Check sheet for the drawn part. Datum: minimum x, y, z corner. Units: mm. A direction names the side the tool comes from. Give positions to 0.01 mm unless a question says otherwise; leave off trailing zeros. Order: outer loops, then holes, each group sorted by start corner. A loop starts at its lowest first (then second) coordinate and runs counter-clockwise, first axis right, second up. Notation, with made-up numbers: M 41.5,-15 L 98.5,-15 A20 cw 98.5,0 Z; hole C 12.25,89.5 d5. An arc over 180 degrees is marked long. Answer as CSV lines item,"result". Start each with the question number.
Q1. Section check C-C, the plane x = 14.25. Record the boundary of the cut face in (y, z).
Q2. Section check B-B, the plane z = 13.5. Record the boundary of the cut face in (x, y).
Q3. Set-up check for the marked faces 1 and 2: record each of +Z, -Z, +X, -X, +Y, -Y from which the full face is reachable in a straight line by a thin tool's end or side.
Q4. Section check A-A, the plane y = 4. Record the boundary of the cut face in (x, z), then the cut area to 3 significant figures.
Q5. Go/stop test with flat-tipped pins: pin 1 (1 mm diameter, centred on x = 8.5, y = 1, fed in from -Z); pin 2 (2 mm diameter, centred on y = 1, z = 8.5, fed in from -X); pin 3 (6 mm diameter, centred on x = 18, y = 10, fed in from -Z); pin 4 (1.6 mm diameter, centred on y = 19, z = 14, fed in from -X). Record where each tip stops, or that it passes through.
Q6. Thickness scan on line 1 (X direction, y = 7.25, z = 56.5); line 2 (X direction, y = 11, z = 83). Record the ranges inside material, lowest first.
Q7. Section check D-D, the plane z = 25. Record the boundary of the cut face in (x, y), then the cut area to 3 significant figures.
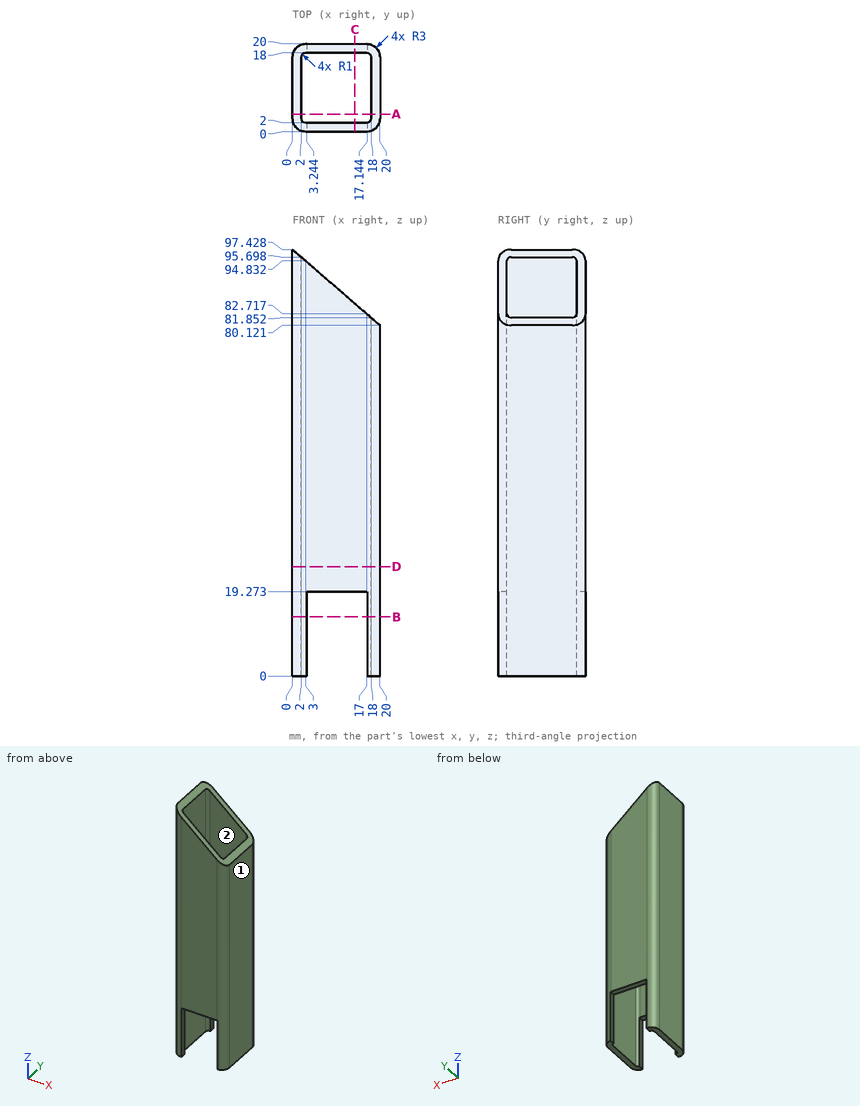
Answer block:
1,outline,"M 0,19.27 L 2,19.27 L 2,85.1 L 0,85.1 Z; M 18,19.27 L 20,19.27 L 20,85.1 L 18,85.1 Z"
2,outline,"M 0,3 A3 ccw 3,0 L 3.24,0 L 3.24,2 L 3,2 A1 cw 2,3 L 2,17 A1 cw 3,18 L 3.24,18 L 3.24,20 L 3,20 A3 ccw 0,17 Z; M 17.14,0 A3 ccw 20,3 L 20,17 A3 ccw 17.14,20 L 17.14,17.99 A1 cw 18,17 L 18,3 A1 cw 17.14,2.01 Z"
3,face 1,"+Z, -Z, +X, +Y, -Y"
3,face 2,"+Z, -Z"
4,outline,"M 0,0 L 2,0 L 2,95.7 L 0,97.43 Z; M 18,0 L 20,0 L 20,80.12 L 18,81.85 Z"
4,area,"355 mm2"
5,pin 1,"stops at z = 19.27"
5,pin 2,"stops at x = 0.17"
5,pin 3,"stops at z = 0"
5,pin 4,"stops at x = 0.25"
6,line 1,"x = 0 to 2, 18 to 20"
6,line 2,"x = 0 to 2"
7,outline,"M 0,3 A3 ccw 3,0 L 17,0 A3 ccw 20,3 L 20,17 A3 ccw 17,20 L 3,20 A3 ccw 0,17 Z; hole M 2,3 A1 ccw 3,2 L 17,2 A1 ccw 18,3 L 18,17 A1 ccw 17,18 L 3,18 A1 ccw 2,17 Z"
7,area,"137 mm2"
